Source: three-view drawing plus pictorial views. Frame: mm from the lowest corner of the part. Give positions to 0.01 mm unless a question says otherwise; leave off trailing zeros. Write each loop counter-clockwise with the first axis right and the second up, starting at its lowest first coordinate (ties: lowest second). Pieces come first, ordered by that corner, then holes.
Q1. Cut plane A-A on x = 76.5. Return the cut outline in (y, z), plus the area to 3 significant figures.
Q2. Line query: L1, parallel to X at y = 82, z = 0.5; L2, parallel to Y at x = 41, z = 6; L3, parallel to Y at x = 77, z = 9. Output: solid intervals per line, ascending.
Q3. Cut plane C-C on z = 3.5. Return the cut outline in (x, y).
Q4. Cut plane D-D on y = 78. Return the cut outline in (x, z), plus the area to 3 significant figures.
Q5. Cut plane B-B on x = 45. Return the cut outline in (y, z), plus the area to 3 significant figures.
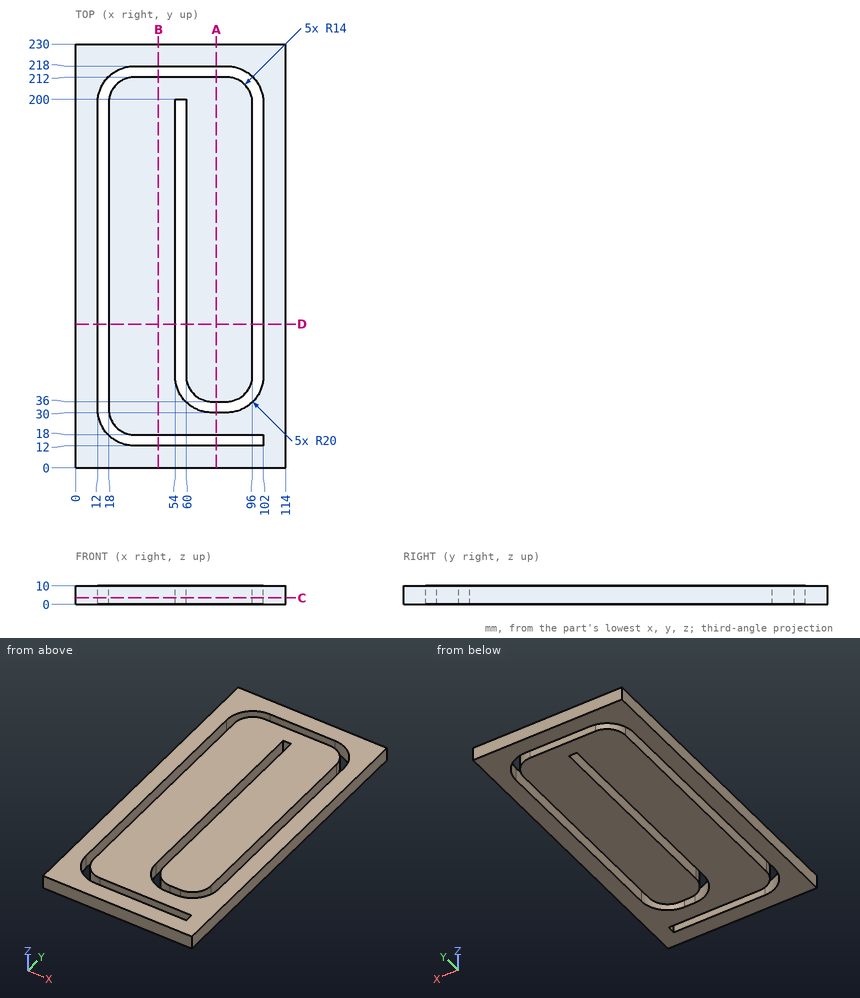
Data:
1. outline: (0, 0) - (12, 0) - (12, 10) - (0, 10) - close; (18, 0) - (30, 0) - (30, 10) - (18, 10) - close; (36, 0) - (212, 0) - (212, 10) - (36, 10) - close; (218, 0) - (230, 0) - (230, 10) - (218, 10) - close
1. area: 2,120 mm2
2. L1: x = 0 to 12, 18 to 54, 60 to 96, 102 to 114
2. L2: y = 0 to 12, 18 to 212, 218 to 230
2. L3: y = 0 to 12, 18 to 30, 36 to 212, 218 to 230
3. outline: (0, 0) - (114, 0) - (114, 230) - (0, 230) - close; hole (12, 32) arc R20 ccw to (32, 12) - (102, 12) - (102, 18) - (32, 18) arc R14 cw to (18, 32) - (18, 198) arc R14 cw to (32, 212) - (82, 212) arc R14 cw to (96, 198) - (96, 50) arc R14 cw to (82, 36) - (74, 36) arc R14 cw to (60, 50) - (60, 200) - (54, 200) - (54, 50) arc R20 ccw to (74, 30) - (82, 30) arc R20 ccw to (102, 50) - (102, 198) arc R20 ccw to (82, 218) - (32, 218) arc R20 ccw to (12, 198) - close
4. outline: (0, 0) - (12, 0) - (12, 10) - (0, 10) - close; (18, 0) - (54, 0) - (54, 10) - (18, 10) - close; (60, 0) - (96, 0) - (96, 10) - (60, 10) - close; (102, 0) - (114, 0) - (114, 10) - (102, 10) - close
4. area: 960 mm2
5. outline: (0, 0) - (12, 0) - (12, 10) - (0, 10) - close; (18, 0) - (212, 0) - (212, 10) - (18, 10) - close; (218, 0) - (230, 0) - (230, 10) - (218, 10) - close
5. area: 2,180 mm2
